Read the model definition and answer for the solid it produces. Units are mm, in the model's axes. Face numbers are marked on the shaded views. Give positions to 0.01 mm unless a question says otherwise; leave off trailing zeros. Write each loop counter-clockwise with the first axis right and the second up, starting at its lowest first coordinate (ties: lowest second). Pieces come first, ordered by that corner, then holes. Notation, with made-up numbers: M 33,58 L 38,58 A24 cw 38,68 Z; hole C 34,-14 d9. An arc over 180 degrees is marked long. Write each question's results on one line, items separated by ' | '. Start each with the question number.
```python
from build123d import *

# Parameters (mm, degrees)
F1_DEPTH = 177.8
F2_DEPTH = 177.8
F3_DEPTH = 203.2
F4_DEPTH = 203.2


with BuildPart() as f1:
    # F0 (on Front) → F1 (new body)
    with BuildSketch(Plane.XZ):
        Polygon((-127, 0), (0, 0), (0, 76.2), align=None)
        Polygon((0, 76.2), (0, 0), (127, 0), align=None)
    extrude(amount=F1_DEPTH)

    # F2 (add): a face of the model
    f2_faces = [f1.faces().sort_by_distance(p)[0] for p in [
        (0, 0, 25.4),
    ]]
    extrude(f2_faces, amount=F2_DEPTH)

    # F0 (on Front) → F3 (join)
    with BuildSketch(Plane.XZ):
        Polygon((0, 101.6), (-203.2, -25.4), (203.2, -25.4), align=None)
        Polygon((127, 0), (0, 0), (-127, 0), (0, 76.2), align=None, mode=Mode.SUBTRACT)
    extrude(amount=F3_DEPTH)

    # F0 (on Front) → F4 (join)
    with BuildSketch(Plane.XZ):
        Polygon((0, 101.6), (-203.2, -25.4), (203.2, -25.4), align=None)
        Polygon((127, 0), (0, 0), (-127, 0), (0, 76.2), align=None, mode=Mode.SUBTRACT)
    extrude(amount=-F4_DEPTH)


solid = f1.part
```
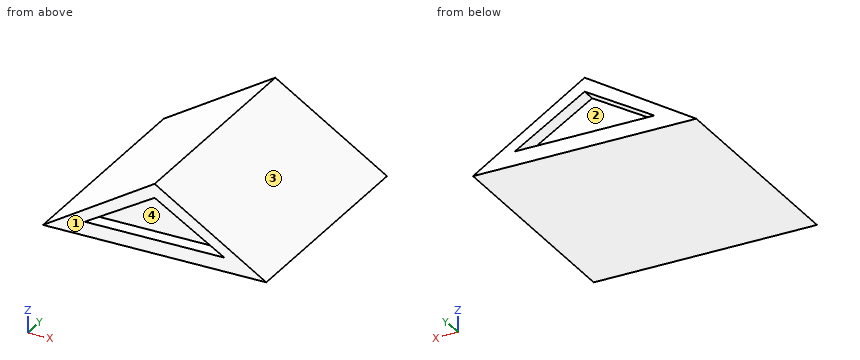
Item 1: Determine the mould class of the marked faces 1, 2, 3 and 4 for opening direction X: +X half, -X half, draft (parallel to the pull), parting line (faces both ways), or undercut.
Item 2: Section C-C, the plane y = 141.5 is taken. Determine the outline of the cut face in (x, z).
Item 3: Section A-A, the plane x = 16 is taken. Determine the outline of the cut face in (y, z), then the cut area to 3 significant figures.
Item 4: Section B-B, the plane z = 34 is taken. Determine the outline of the cut face in (x, y), then the cut area to 3 significant figures.
Item 5: Given P1, Ø20.5, axis at x = 17.5, y = 187.5, coming from the +Z side; P2, Ø23, axis at x = 3.5, z = 23, coming from the +Y side; P3, Ø1.5, axis at x = -45, z = 27.5, coming from the -Y side, each flat-ended and moving along its own axis, determine where each tip first touches the part or whether it passes through.
Item 6: Straight lines are drawn through the part: line 1 (Y direction, x = 7.5, z = 20); line 2 (Z direction, x = -161, y = 136) (3 decimals); line 3 (Z direction, x = -143.5, y = 44). For each, find the intervals that lie inside material, in ascending order.
Item 7: Section D-D, the plane z = -13 is taken. Determine the outline of the cut face in (x, y).
Worked out:
1) face 1: draft | face 2: undercut | face 3: +X half | face 4: undercut
2) outline: M -203.2,-25.4 L 203.2,-25.4 L 0,101.6 Z
3) outline: M -203.2,-25.4 L 203.2,-25.4 L 203.2,0 L 177.8,0 L 177.8,66.6 L 203.2,66.6 L 203.2,91.6 L -203.2,91.6 L -203.2,66.6 L -177.8,66.6 L -177.8,0 L -203.2,0 Z | area: 44,200 mm²
4) outline: M -108.16,-203.2 L -70.33,-203.2 L -70.33,-177.8 L 70.33,-177.8 L 70.33,-203.2 L 108.16,-203.2 L 108.16,203.2 L 70.33,203.2 L 70.33,177.8 L -70.33,177.8 L -70.33,203.2 L -108.16,203.2 Z | area: 80,800 mm²
5) P1: stops at z = 97.07 | P2: stops at y = 177.8 | P3: stops at y = -177.8
6) line 1: y = -177.8 to 177.8 | line 2: z = -25.4 to 0.975 | line 3: z = -25.4 to 11.91
7) outline: M -183.36,-203.2 L 183.36,-203.2 L 183.36,203.2 L -183.36,203.2 Z
